```python
from build123d import *

# Parameters (mm, degrees)
F0_W     = 25.4
F0_H     = 25.4
F1_DEPTH = 38.1
F1_TAPER = -40
F2_W     = 74.0993918957
F2_H     = 74.0993918957
F3_DEPTH = 73.66
F3_TAPER = 20


with BuildPart() as f1:
    # F0 (on Top) → F1 (new body)
    with BuildSketch(Plane.XY):
        with Locations((0, -12.7)):
            Rectangle(F0_W, F0_H)
    extrude(amount=F1_DEPTH, taper=F1_TAPER)

    # F2 (on face) → F3 (join)
    with BuildSketch(Plane.XY.offset(38.1)):
        with Locations((0, -12.7)):
            Rectangle(F2_W, F2_H)
    extrude(amount=F3_DEPTH, taper=F3_TAPER)


solid = f1.part
```
Geometry check sheet. Reference: the model listing, model coordinates, mm. A direction names the side the tool comes from. Give positions to 0.01 mm unless a question says otherwise; leave off trailing zeros. Write each loop counter-clockwise with the first axis right and the second up, starting at its lowest first coordinate (ties: lowest second). Pieces come first, ordered by that corner, then holes. Notation, with made-up numbers: (16.5, 22) -> (29.5, 22) arc R28 cw to (29.5, 56) -> close; hole circle Ø7 at (-28.75, -32). An arc over 180 degrees is marked (long way). Use one line per item in the form item = value.
Item 1: Depth check by flat-ended pin: pin 1 Ø10 at (x, z) = (28.5, 53) entering from +Y; pin 2 Ø2 at (x, z) = (-22.5, 44.5) entering from -Y; pin 3 Ø12 at (y, z) = (12, 26.5) entering from +X; pin 4 Ø8 at (y, z) = (21, 63) entering from -X. Enter the tip coordinate at first touch or a pass-through.
Results list:
pin_1 = 20.75
pin_2 = -47.78
pin_3 = 39.97
pin_4 = through
Item 2: Sectioned sample at A-A on z = 60. Enter the section's corners in (x, y).
Results list:
outline = (-29.08, -41.78) -> (29.08, -41.78) -> (29.08, 16.38) -> (-29.08, 16.38) -> close
Item 3: Sectioned sample at B-B on z = 47. Enter the section's corners in (x, y), plus the area to 3 significant figures.
Results list:
outline = (-33.81, -46.51) -> (33.81, -46.51) -> (33.81, 21.11) -> (-33.81, 21.11) -> close
area = 4,570 mm2
Item 4: Scan lines: line 1 (Z direction, x = -4, y = 28.5); line 2 (X direction, y = -6.5, z = 6.5); line 3 (X direction, y = -33.5, z = 78). Record each from-to range of solid material in increasing order.
Results list:
line_1 = 33.96 to 38.1
line_2 = -18.15 to 18.15
line_3 = -22.53 to 22.53
Item 5: Access from +Z, -Z, +X, -X, +Y, -Y to the whole of each face (thin tool, end or side, straight path). Record for faces 1 (the flat face through (0, -52, 38.1)), 2 (the flat face through (0, -13, 0)).
Results list:
face_1 = +Z
face_2 = -Z, +X, -X, +Y, -Y
